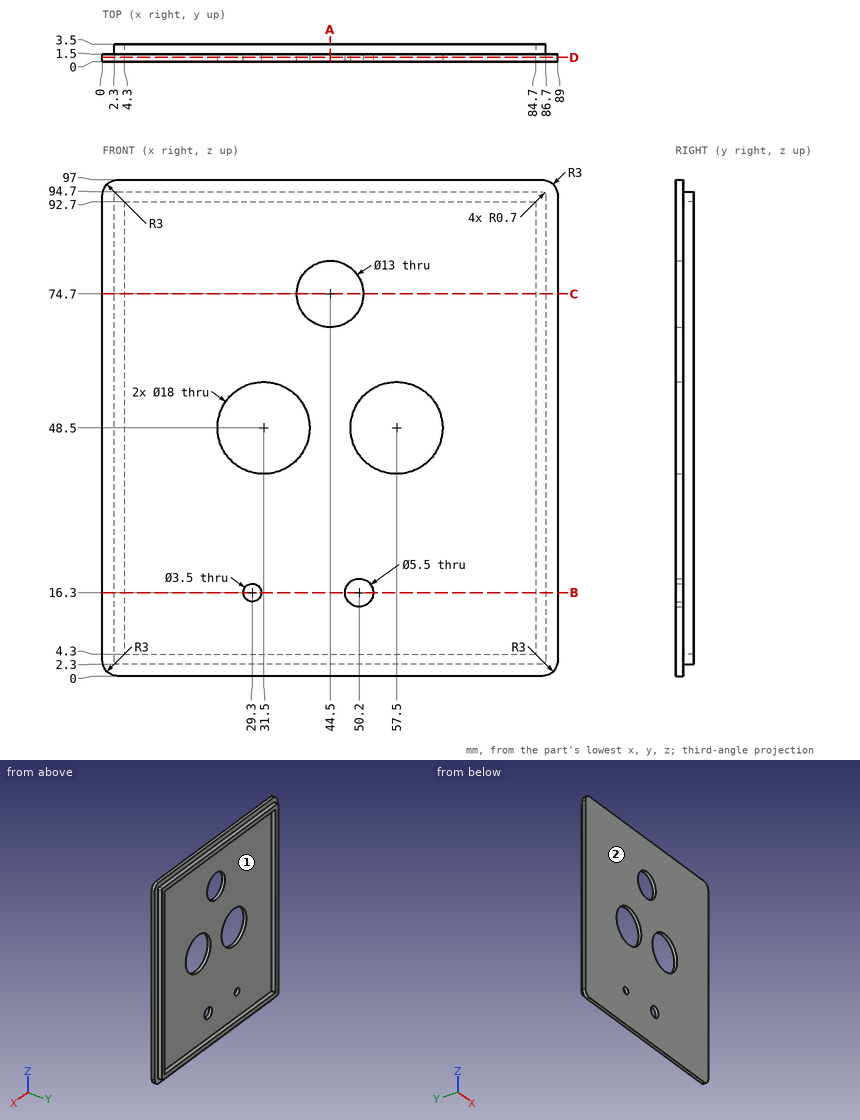
Could you check a few things on this drawing? It's one solid part, dimensions in mm from its lowest x, y, z. Coordinates: 2 decimals unless noted, no trailing zeros. Order: outer loops, then holes, each group sorted by start corner. A loop starts at its lowest first (then second) coordinate and runs counter-clockwise, first axis right, second up.
1) We'd pull the mould along X, two halves only. Please class the marked faces 1 and 2: +X half, -X half, draft (parallel to the pull), parting line (faces both ways), or undercut.
2) Imagine slicing it at B-B on z = 16.3. List the corners of the cut face in (x, y) for me, and give its area (3 significant figures).
3) Will these pins go through, and if not, where does the flat tip stop? pin 1 (2 mm diameter, centred on y = 2, z = 69, fed in from -X); pin 2 (3.5 mm diameter, centred on x = 50.2, z = 16.3, fed in from -Y); pin 3 (0.6 mm diameter, centred on x = 46.5, y = 2.5, fed in from +Z); pin 4 (0.6 mm diameter, centred on y = 2, z = 38.5, fed in from +X).
4) Imagine slicing it at C-C on z = 74.7. List the corners of the cut face in (x, y) for me, and give its area (3 significant figures).
5) I need wall thicknesses on line 1 (X direction, y = 0.8, z = 16.3); line 2 (X direction, y = 0.5, z = 48.5); line 3 (Z direction, x = 49, y = 2.85). Which ranges of each line are inside material? Lowest first, please.
6) Imagine slicing it at D-D on y = 0.9. List the corners of the cut face in (x, z) for me, and give its area (3 significant figures).
7) Imagine slicing it at A-A on x = 44.5. List the corners of the cut face in (y, z) for me.
Response values:
1. face 1: undercut
1. face 2: draft
2. outline: (0, 0) - (27.55, 0) - (27.55, 1.5) - (4.3, 1.5) - (4.3, 3.5) - (2.3, 3.5) - (2.3, 1.5) - (0, 1.5) - close; (31.05, 0) - (47.45, 0) - (47.45, 1.5) - (31.05, 1.5) - close; (52.95, 0) - (89, 0) - (89, 1.5) - (86.7, 1.5) - (86.7, 3.5) - (84.7, 3.5) - (84.7, 1.5) - (52.95, 1.5) - close
2. area: 128 mm2
3. pin 1: stops at x = 0
3. pin 2: passes through
3. pin 3: stops at z = 94.7
3. pin 4: stops at x = 86.7
4. outline: (0, 0) - (38, 0) - (38, 1.5) - (4.3, 1.5) - (4.3, 3.5) - (2.3, 3.5) - (2.3, 1.5) - (0, 1.5) - close; (51, 0) - (89, 0) - (89, 1.5) - (86.7, 1.5) - (86.7, 3.5) - (84.7, 3.5) - (84.7, 1.5) - (51, 1.5) - close
4. area: 122 mm2
5. line 1: x = 0 to 27.55, 31.05 to 47.45, 52.95 to 89
5. line 2: x = 0 to 22.5, 40.5 to 48.5, 66.5 to 89
5. line 3: z = 2.3 to 4.3, 92.7 to 94.7
6. outline: (0, 3) arc R3 ccw to (3, 0) - (86, 0) arc R3 ccw to (89, 3) - (89, 94) arc R3 ccw to (86, 97) - (3, 97) arc R3 ccw to (0, 94) - close; hole circle Ø18 at (31.5, 48.5); hole circle Ø3.5 at (29.3, 16.3); hole circle Ø13 at (44.5, 74.7); hole circle Ø5.5 at (50.2, 16.3); hole circle Ø18 at (57.5, 48.5)
6. area: 7,950 mm2
7. outline: (0, 0) - (1.5, 0) - (1.5, 2.3) - (3.5, 2.3) - (3.5, 4.3) - (1.5, 4.3) - (1.5, 68.2) - (0, 68.2) - close; (0, 81.2) - (1.5, 81.2) - (1.5, 92.7) - (3.5, 92.7) - (3.5, 94.7) - (1.5, 94.7) - (1.5, 97) - (0, 97) - close
